Here's how the part is built. I have some questions about the finished solid (model axes, mm). Coordinates: 2 decimals unless noted, no trailing zeros. Loops run counter-clockwise (first coordinate to the right, second up) from the corner with the lowest first, then second, coordinate; pieces in that order, holes last.
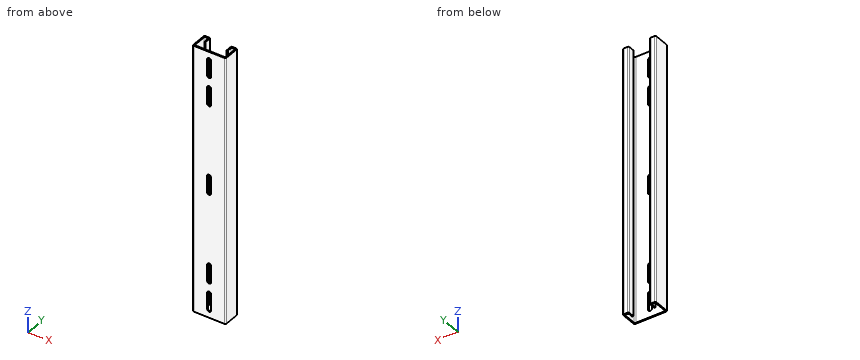
from build123d import *

# Parameters (mm, degrees)
EXTRUDE_1_DEPTH     = 330
CUT_EXTRUDE_1_DEPTH = 331.802811354


with BuildPart() as part:
    # 草图1 → 凸台-拉伸1 (new body)
    with BuildSketch(Plane.XY):
        with BuildLine():
            Line((-19, 10.5), (-14.5, 10.5))
            ThreePointArc((-14.5, 10.5), (-13.439339828, 10.060660172), (-13, 9))
            Line((-13, 9), (-13, 2))
            Line((-13, 2), (-14.5, 2))
            Line((-14.5, 2), (-14.5, 7.5))
            ThreePointArc((-14.5, 7.5), (-14.939339828, 8.560660172), (-16, 9))
            Line((-16, 9), (-17.5, 9))
            ThreePointArc((-17.5, 9), (-18.560660172, 8.560660172), (-19, 7.5))
            Line((-19, 7.5), (-19, -7.5))
            ThreePointArc((-19, -7.5), (-18.560660172, -8.560660172), (-17.5, -9))
            Line((-17.5, -9), (17.5, -9))
            ThreePointArc((17.5, -9), (18.560660172, -8.560660172), (19, -7.5))
            Line((19, -7.5), (19, 7.5))
            ThreePointArc((19, 7.5), (18.560660172, 8.560660172), (17.5, 9))
            Line((17.5, 9), (16, 9))
            ThreePointArc((16, 9), (14.939339828, 8.560660172), (14.5, 7.5))
            Line((14.5, 7.5), (14.5, 2))
            Line((14.5, 2), (13, 2))
            Line((13, 2), (13, 9))
            ThreePointArc((13, 9), (13.439339828, 10.060660172), (14.5, 10.5))
            Line((14.5, 10.5), (19, 10.5))
            ThreePointArc((19, 10.5), (20.060660172, 10.060660172), (20.5, 9))
            Line((20.5, 9), (20.5, -9))
            ThreePointArc((20.5, -9), (20.060660172, -10.060660172), (19, -10.5))
            Line((19, -10.5), (-19, -10.5))
            ThreePointArc((-19, -10.5), (-20.060660172, -10.060660172), (-20.5, -9))
            Line((-20.5, -9), (-20.5, 9))
            ThreePointArc((-20.5, 9), (-20.060660172, 10.060660172), (-19, 10.5))
        make_face()
    extrude(amount=EXTRUDE_1_DEPTH)

    # 草图3 → 切除-拉伸1 (cut, through all)
    with BuildSketch(Plane(origin=(0, 0, 0), x_dir=(1, 0, 0), z_dir=(0, 1, 0))):
        with BuildLine():
            Line((2.5, -10), (2.5, -30))
            ThreePointArc((2.5, -30), (0, -32.5), (-2.5, -30))
            Line((-2.5, -30), (-2.5, -10))
            ThreePointArc((-2.5, -10), (0, -7.5), (2.5, -10))
        make_face()
        with BuildLine():
            Line((2.5, -45), (2.5, -65))
            ThreePointArc((2.5, -65), (0, -67.5), (-2.5, -65))
            Line((-2.5, -65), (-2.5, -45))
            ThreePointArc((-2.5, -45), (0, -42.5), (2.5, -45))
        make_face()
        with BuildLine():
            Line((2.5, -155), (2.5, -175))
            ThreePointArc((2.5, -175), (0, -177.5), (-2.5, -175))
            Line((-2.5, -175), (-2.5, -155))
            ThreePointArc((-2.5, -155), (0, -152.5), (2.5, -155))
        make_face()
        with BuildLine():
            Line((-2.5, -320), (-2.5, -300))
            ThreePointArc((-2.5, -300), (0, -297.5), (2.5, -300))
            Line((2.5, -300), (2.5, -320))
            ThreePointArc((2.5, -320), (0, -322.5), (-2.5, -320))
        make_face()
        with BuildLine():
            Line((-2.5, -285), (-2.5, -265))
            ThreePointArc((-2.5, -265), (0, -262.5), (2.5, -265))
            Line((2.5, -265), (2.5, -285))
            ThreePointArc((2.5, -285), (0, -287.5), (-2.5, -285))
        make_face()
    extrude(amount=-CUT_EXTRUDE_1_DEPTH, mode=Mode.SUBTRACT)


solid = part.part
Q1. Suppose I cut it at B-B on z = 181. Write out the boundary of the cut face in (x, y).
Q2. Please list where these lines run through material, in increasing order: probe 1 along X at (y, z) = (5.5, 268.5); probe 2 along X at (y, z) = (-5.75, 216); probe 3 along Y at (x, z) = (-16, 180).
Q3. Suppose I cut it at A-A on y = -2.25. Write out the boundary of the cut face in (x, z).
Q4. Suppose I cut it at D-D on x = -8. Write out the boundary of the cut face in (y, z), and give its area (3 significant figures).
Q5. Will these pins go through, and if not, where does the flat tip stop? P1, Ø10, axis at x = -11.5, y = 7.5, coming from the -Z side; P2, Ø1.6, axis at y = -10, z = 164.5, coming from the -X side; P3, Ø0.8, axis at y = -10, z = 169.5, coming from the +X side; P4, Ø0.8, axis at y = -10, z = 306.5, coming from the -X side.
Check values:
1. outline: (-20.5, -9) arc R1.5 ccw to (-19, -10.5) - (19, -10.5) arc R1.5 ccw to (20.5, -9) - (20.5, 9) arc R1.5 ccw to (19, 10.5) - (14.5, 10.5) arc R1.5 ccw to (13, 9) - (13, 2) - (14.5, 2) - (14.5, 7.5) arc R1.5 cw to (16, 9) - (17.5, 9) arc R1.5 cw to (19, 7.5) - (19, -7.5) arc R1.5 cw to (17.5, -9) - (-17.5, -9) arc R1.5 cw to (-19, -7.5) - (-19, 7.5) arc R1.5 cw to (-17.5, 9) - (-16, 9) arc R1.5 cw to (-14.5, 7.5) - (-14.5, 2) - (-13, 2) - (-13, 9) arc R1.5 ccw to (-14.5, 10.5) - (-19, 10.5) arc R1.5 ccw to (-20.5, 9) - close
2. probe 1: x = -20.5 to -19, -14.5 to -13, 13 to 14.5, 19 to 20.5
2. probe 2: x = -20.5 to -19, 19 to 20.5
2. probe 3: y = -10.5 to -9, 9 to 10.5
3. outline: (-20.5, 0) - (-19, 0) - (-19, 330) - (-20.5, 330) - close; (19, 0) - (20.5, 0) - (20.5, 330) - (19, 330) - close
4. outline: (-10.5, 0) - (-9, 0) - (-9, 330) - (-10.5, 330) - close
4. area: 495 mm2
5. P1: stops at z = 0
5. P2: stops at x = -20.49
5. P3: stops at x = 20.37
5. P4: stops at x = -20.37
